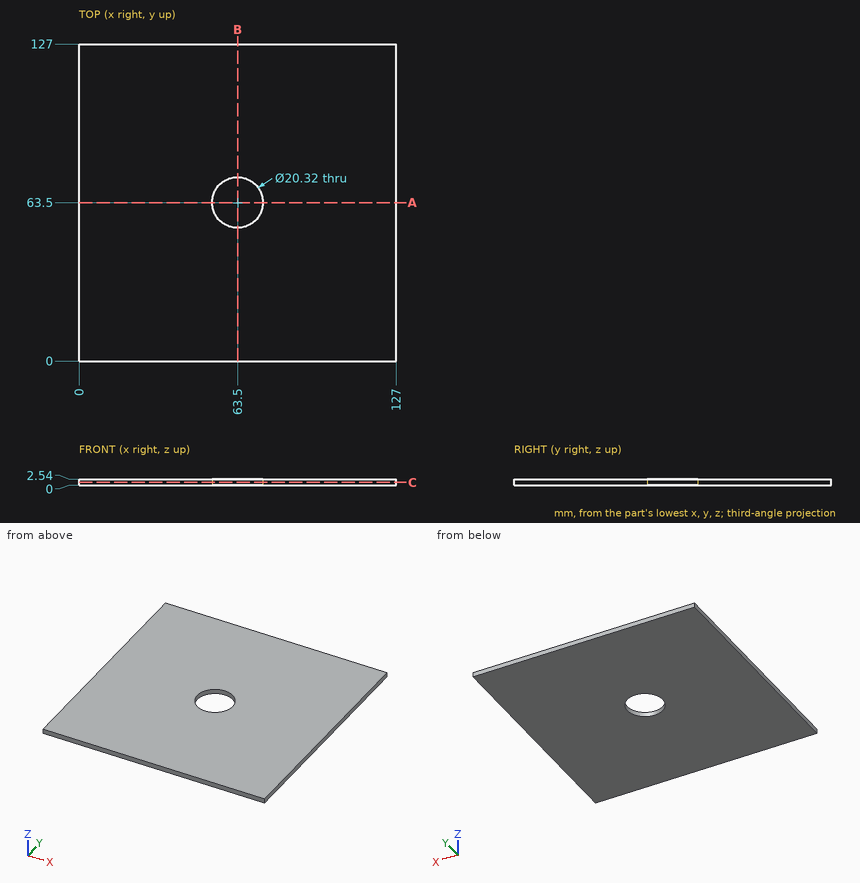
Design review of the part shown in the three views and the two pictorial views. Dimensions are in mm from the part's minimum x, y and z. Round coordinates to 2 decimals unless told otherwise and drop trailing zeros. Loops run counter-clockwise (first coordinate to the right, second up) from the corner with the lowest first, then second, coordinate; pieces in that order, holes last. Notation, with made-up numbers: (-39.5, 40.25) -> (-33.5, 40.25) arc R30 cw to (-33.5, 68.25) -> close; hole circle Ø6 at (-1.5, -5.5). An arc over 180 degrees is marked (long way). Answer as a JSON object with one key per item and string values. Group by question number.
1) We need section A-A on y = 63.5. Write out the cut boundary in (x, z), then the cut area to 3 significant figures.
2) For line 1 (Y direction, x = 63.5, z = 0.85); line 2 (X direction, y = 63, z = 1.75); line 3 (X direction, y = 60.5, z = 1.3), list the stretches that pass through material, from the lowest coordinate up. Write a range as [from, to].
3) For pin 1 Ø1 at (x, z) = (14, 0.5) entering from -Y, flat-tipped, find the tip position at first contact; note if it passes through.
4) We need section C-C on z = 1.2. Write out the cut boundary in (x, y), then the cut area to 3 significant figures.
Result set:
{
 "1": {"outline": "(0, 0) -> (53.34, 0) -> (53.34, 2.54) -> (0, 2.54) -> close; (73.66, 0) -> (127, 0) -> (127, 2.54) -> (73.66, 2.54) -> close", "area": "271 mm²"},
 "2": {"line 1": "[0, 53.34], [73.66, 127]", "line 2": "[0, 53.35], [73.65, 127]", "line 3": "[0, 53.79], [73.21, 127]"},
 "3": {"pin 1": "y = 0"},
 "4": {"outline": "(0, 0) -> (127, 0) -> (127, 127) -> (0, 127) -> close; hole circle Ø20.32 at (63.5, 63.5)", "area": "15,800 mm²"}
}
